Autodesk Inventor part; units mm, degrees
ref_plane "YZ Plane" through (0, 0, 0) normal (1, 0, 0) x (0, 1, 0)
ref_plane "XZ Plane" through (0, 0, 0) normal (0, 1, 0) x (-1, 0, 0)
ref_plane "XY Plane" through (0, 0, 0) normal (0, 0, 1) x (1, 0, 0)
sketch "Sketch1" plane through (0, 0, 0) normal (0, 0, 1) x (1, 0, 0)
  line L0 (0, 0) -> (0, 68.58)
  line L1 (0, 68.58) -> (40.64, 68.58)
  line L2 (40.64, 30.48) -> (6.35, 0)
  line L3 (6.35, 0) -> (0, 0)
  line L4 (40.64, 68.58) -> (40.64, 30.48)
  dimension "d1" = 40.64
  dimension "d2" = 6.35
  dimension "d6" = 90
  dimension "d21" = 38.1
  dimension "d22" = 30.48
revolve "Revolution1" add sketch "Sketch1" angle 360 about axis through (0, 0, 0) along (0, 1, 0)
shell "Shell1" thickness 1.5 outward yes removed faces 2 at (-10.0721, 68.58, 13.6928) at (-1.8127, 0, 0.4771)
sketch "Sketch2" plane through (0, 0, 0) normal (0, -1, 0) x (1, 0, 0)
  line L0 (6.2865, -0.8255) -> (7.9502, -0.8255)
  line L1 (7.9502, -0.8255) -> (7.9502, 0.8255)
  line L2 (7.9502, 0.8255) -> (6.2865, 0.8255)
  line L3 (6.2865, 0.8255) -> (6.2865, -0.8255)
  line L4 (6.2865, -0.8255) -> (7.9502, 0.8255) construction
  line L5 (7.9502, -0.8255) -> (6.2865, 0.8255) construction
  line L6 (0, 1.1822) -> (0, -1.5875) construction
  line L7 (-6.2865, -0.8255) -> (-7.9502, -0.8255)
  line L8 (-7.9502, -0.8255) -> (-7.9502, 0.8255)
  line L9 (-7.9502, 0.8255) -> (-6.2865, 0.8255)
  line L10 (-6.2865, 0.8255) -> (-6.2865, -0.8255)
  line L11 (2.1925, 0) -> (-0.3475, 0) construction
  line L12 (-0.8255, 6.2865) -> (0.8255, 6.2865)
  line L13 (0.8255, 6.2865) -> (0.8255, 7.9502)
  line L14 (0.8255, 7.9502) -> (-0.8255, 7.9502)
  line L15 (-0.8255, 7.9502) -> (-0.8255, 6.2865)
  line L16 (-0.8255, 6.2865) -> (0.8255, 7.9502) construction
  line L17 (0.8255, 6.2865) -> (-0.8255, 7.9502) construction
  line L18 (-0.8255, -6.2865) -> (0.8255, -6.2865)
  line L19 (0.8255, -6.2865) -> (0.8255, -7.9502)
  line L20 (0.8255, -7.9502) -> (-0.8255, -7.9502)
  line L21 (-0.8255, -7.9502) -> (-0.8255, -6.2865)
  line L22 (-0.8255, -6.2865) -> (0.8255, -7.9502) construction
  line L23 (0.8255, -6.2865) -> (-0.8255, -7.9502) construction
  circle A0 centre (0, 0) radius 6.35
  point P0 (0, 0)
  point P1 (7.1183, 0)
  point P2 (-7.1183, 0)
  point P3 (0, 7.1183)
  point P4 (0, -7.1183)
  dimension "d8" = 1.651
  dimension "d9" = 1.6637
  dimension "d11" = 1.6637
  dimension "d12" = 1.651
  dimension "d17" = 0.0635
  dimension "d18" = 0.0635
extrude "Extrusion3" cut sketch "Sketch2" against normal blind 1.651 contours L3 L2 A0 L0 | A0 L2 L1 L0 | A0 L21 L18 L19 | L19 L20 L21 A0 | A0 L15 L14 L13 | L13 L12 L15 A0 | A0 L9 L10 L7 | L7 L8 L9 A0
equation "\"BendRadius\" = Thickness"
equation "\"BendReliefWidth\" = Thickness"
equation "\"BendReliefDepth\" = 0.5 * Thickness"
equation "\"CornerReliefSize\" = 4 * Thickness"
equation "\"MinimumRemnant\" = 2 * Thickness"
equation "\"TransitionRadius\" = BendRadius"
equation "\"JacobiRadiusSize\" = BendRadius"
equation "\"GapSize\" = Thickness"
properties part number "LargerWidefieldCone_v3"
Design review of the part built by this model. Coordinates are the model's own, in mm. Round coordinates to 2 decimals unless told otherwise and drop trailing zeros. Write each loop counter-clockwise with the first axis right and the second up, starting at its lowest first coordinate (ties: lowest second). Pieces come first, ordered by that corner, then holes. Notation, with made-up numbers: (4.5, 17) -> (13.5, 17) arc R17 ccw to (13.5, 47) -> close; hole circle Ø7 at (-14.75, -33.75). An arc over 180 degrees is marked (long way). One line per item, written item: value. Start each with the question number.
Q1. The part is to be moulded in two halves that separate along Z. For faces 1 (the face through (-5.291, 49.263, 40.294)), 2 (the face through (11.737, 5.293, -3.696)), 3 (the face through (-3, 0, 6)), 4 (the face through (10.211, 1.865, -3.216)), say which applies: pulls with the +Z half, pulls with the -Z half, needs draft (parallel to the pull), parting line crosses it, or undercut.
Q2. Add section B-B (y = 17). Give the boundary of the cut face in (x, z) (3 decimals), then the cut area to 3 significant figures.
Q3. Insertion check: P1, Ø1.6, axis at y = 1, z = 7.5, coming from the +X side; P2, Ø5, axis at y = 33.5, z = 3.5, coming from the -X side; P3, Ø12, axis at x = -17, y = 49, coming from the -Z side; P4, Ø12, axis at x = 30.5, y = 8.5, coming from the +Z side. Each pin has a flat end and moves straight along its axis. Give the tip position at first contact, or say it passes through.
Q4. Add section A-A (y = 57). Give the boundary of the cut face in (x, z).
Q5. To check wall thickness, follow probe 1 along Z at (x, y) = (0, 56); probe 2 along X at (y, z) = (53, -23.5); probe 3 along Z at (x, y) = (2, 21.5). State the ranges of each line that lie inside material, in increasing order.
Response:
1. face 1: undercut
1. face 2: undercut
1. face 3: needs draft
1. face 4: parting line crosses it
2. outline: circle Ø55.466 at (0, 0); hole circle Ø50.95 at (0, 0)
2. area: 377 mm^2
3. P1: stops at x = 7.75
3. P2: stops at x = -42.13
3. P3: stops at z = -40.68
3. P4: passes through
4. outline: circle Ø84.28 at (0, 0); hole circle Ø81.28 at (0, 0)
5. probe 1: z = -42.14 to -40.64, 40.64 to 42.14
5. probe 2: x = -34.98 to -33.16, 33.16 to 34.98
5. probe 3: z = -32.73 to -30.47, 30.47 to 32.73
